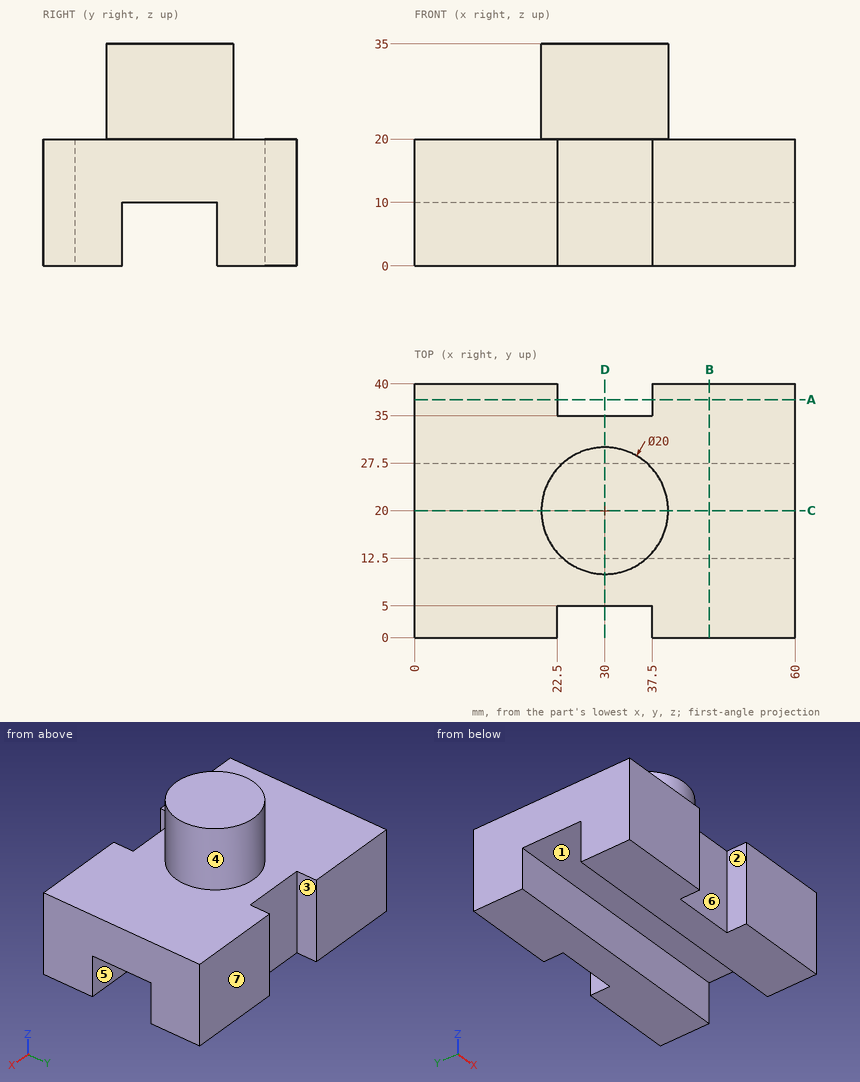
Source: three-view drawing plus pictorial views. Frame: mm from the lowest corner of the part. A direction names the side the tool comes from. Coordinates: 2 decimals unless noted, no trailing zeros. Order: outer loops, then holes, each group sorted by start corner. A loop starts at its lowest first (then second) coordinate and runs counter-clockwise, first axis right, second up. Notation, with made-up numbers: M -20.75,37.5 L 23.25,37.5 A14 ccw 23.25,61.5 Z; hole C 5.25,28 d7. An arc over 180 degrees is marked long. Answer in a Markdown table with one row per item.
(1) Material intervals for line 1 (Y direction, x = 28, z = 9); line 2 (Y direction, x = 11.5, z = 5); line 3 (Y direction, x = 31.5, z = 10.5), sorted ascending. Write a range as [from, to].
Numbers:
| item | result |
|---|---|
| line 1 | y = [5, 12.5], [27.5, 35] |
| line 2 | y = [0, 12.5], [27.5, 40] |
| line 3 | y = [5, 35] |
(2) Contact query for flat-ended pins moving along their axis: pin 1 Ø4.5 at (x, z) = (33, 11) entering from -Y; pin 2 Ø6 at (x, z) = (21, 29.5) entering from -Y; pin 3 Ø2 at (y, z) = (11.5, 23) entering from -X. Output: stop coordinate, or through.
Numbers:
| item | result |
|---|---|
| pin 1 | stops at y = 5 |
| pin 2 | stops at y = 12 |
| pin 3 | stops at x = 23.39 |
(3) Access query for the marked faces 1, 2, 3 and 4. Directions: +Z, -Z, +X, -X, +Y, -Y. A direction counts if a zero-diameter tool reaches every point of the face in a straight line with its end or side. Return the directions, or none.
Numbers:
| item | result |
|---|---|
| face 1 | -Z, +X, -X |
| face 2 | +Z, -Z, -Y |
| face 3 | +Z, -Z, +Y |
| face 4 | +Z |
(4) Section query A-A, the plane y = 37.5. Output: boundary loops of the cut face in (x, z), plus the area to 3 significant figures.
Numbers:
| item | result |
|---|---|
| outline | M 0,0 L 22.5,0 L 22.5,20 L 0,20 Z; M 37.5,0 L 60,0 L 60,20 L 37.5,20 Z |
| area | 900 mm^2 |
(5) Section query D-D, the plane x = 30. Output: boundary loops of the cut face in (y, z), plus the area to 3 significant figures.
Numbers:
| item | result |
|---|---|
| outline | M 5,0 L 12.5,0 L 12.5,10 L 27.5,10 L 27.5,0 L 35,0 L 35,20 L 30,20 L 30,35 L 10,35 L 10,20 L 5,20 Z |
| area | 750 mm^2 |
(6) Section query B-B, the plane x = 46.5. Output: boundary loops of the cut face in (y, z).
Numbers:
| item | result |
|---|---|
| outline | M 0,0 L 12.5,0 L 12.5,10 L 27.5,10 L 27.5,0 L 40,0 L 40,20 L 0,20 Z |
(7) Section query C-C, the plane y = 20. Output: boundary loops of the cut face in (x, z).
Numbers:
| item | result |
|---|---|
| outline | M 0,10 L 60,10 L 60,20 L 40,20 L 40,35 L 20,35 L 20,20 L 0,20 Z |
(8) Draft query along Y for the marked faces 5, 6 and 7. Return one class per face: pulls with the +Y half, pulls with the -Y half, needs draft (parallel to the pull), parting line crosses it, or undercut.
Numbers:
| item | result |
|---|---|
| face 5 | undercut |
| face 6 | pulls with the -Y half |
| face 7 | pulls with the +Y half |
